```python
from build123d import *

# Parameters (mm, degrees)
SKETCH1_R           = 2.5
BOSS_EXTRUDE1_DEPTH = 6


with BuildPart() as part:
    # Sketch1 → Boss-Extrude1 (new body)
    with BuildSketch(Plane.XY):
        Polygon((140, 0), (0, 0), (0, -9), (-7, -9), (-7, -29), (0, -29), (0, -47.27), (140, -47.27), (140, -29), (147, -29), (147, -9), (140, -9), align=None)
        with Locations((120, -19)):
            Circle(SKETCH1_R, mode=Mode.SUBTRACT)
        with Locations((20, -19)):
            Circle(SKETCH1_R, mode=Mode.SUBTRACT)
        with BuildLine():
            Line((45, -34), (95, -34))
            ThreePointArc((95, -34), (110, -19), (95, -4))
            Line((95, -4), (45, -4))
            ThreePointArc((45, -4), (30, -19), (45, -34))
        make_face(mode=Mode.SUBTRACT)
    extrude(amount=BOSS_EXTRUDE1_DEPTH)


solid = part.part
```
Model file for the job. Use its own axes, mm. A direction names the side the tool comes from. Round coordinates to 2 decimals unless told otherwise and drop trailing zeros. Order: outer loops, then holes, each group sorted by start corner. A loop starts at its lowest first (then second) coordinate and runs counter-clockwise, first axis right, second up. Notation, with made-up numbers: M 73,62.5 L 132,62.5 A30 ccw 132,93.5 Z; hole C 57,48.5 d6. An arc over 180 degrees is marked long. Use CSV: the item, a comma, the result in double quotes.
Item 1: Which spindle directions (+Z, -Z, +X, -X, +Y, -Y) get a long thin tool onto all of the face, cutting with end or side? Do faces 4 (the face through (144, -9, 3)), 5 (the face through (-4, -29, 3)), 6 (the face through (140, -38, 3)), 7 (the face through (30, -19, 3)). Say none if no direction does.
Worked answers:
face 4,"+Z, -Z, +X, +Y"
face 5,"+Z, -Z, -X, -Y"
face 6,"+Z, -Z, +X, -Y"
face 7,"+Z, -Z"
Item 2: Saw through at B-B (y = -19). List the corners of the cut face in (x, z).
Worked answers:
outline,"M -7,0 L 17.5,0 L 17.5,6 L -7,6 Z; M 22.5,0 L 30,0 L 30,6 L 22.5,6 Z; M 110,0 L 117.5,0 L 117.5,6 L 110,6 Z; M 122.5,0 L 147,0 L 147,6 L 122.5,6 Z"
Item 3: Pin check, flat tips, straight feed: pin 1 (1.8 mm diameter, centred on x = -4, z = 3.5, fed in from +Y); pin 2 (1.8 mm diameter, centred on y = -41.5, z = 2, fed in from -X); pin 3 (3 mm diameter, centred on x = -3, z = 2.5, fed in from -Y). Stop position of each tip, or through.
Worked answers:
pin 1,"y = -9"
pin 2,"x = 0"
pin 3,"y = -29"
Item 4: Saw through at C-C (z = 1.5). List the corners of the cut face in (x, y).
Worked answers:
outline,"M -7,-29 L 0,-29 L 0,-47.27 L 140,-47.27 L 140,-29 L 147,-29 L 147,-9 L 140,-9 L 140,0 L 0,0 L 0,-9 L -7,-9 Z; hole C 20,-19 d5; hole M 45,-34 L 95,-34 A15 ccw 95,-4 L 45,-4 A15 ccw Z; hole C 120,-19 d5"
Item 5: Probe probe 1 along Y at (x, z) = (120, 2.15); probe 2 along X at (y, z) = (-18, 0.7); probe 3 along Y at (x, z) = (93, 1). List the from-to ranges inside material, lowest first.
Worked answers:
probe 1,"-47.27 to -21.5, -16.5 to 0"
probe 2,"-7 to 17.71, 22.29 to 30.03, 109.97 to 117.71, 122.29 to 147"
probe 3,"-47.27 to -34, -4 to 0"
Item 6: Saw through at A-A (x = 89.5). List the corners of the cut face in (y, z), plus the area to 3 significant figures.
Worked answers:
outline,"M -47.27,0 L -34,0 L -34,6 L -47.27,6 Z; M -4,0 L 0,0 L 0,6 L -4,6 Z"
area,"104 mm²"
Item 7: Saw through at D-D (y = -25.5). List the corners of the cut face in (x, z).
Worked answers:
outline,"M -7,0 L 31.48,0 L 31.48,6 L -7,6 Z; M 108.52,0 L 147,0 L 147,6 L 108.52,6 Z"
Item 8: Pull direction Y, two halves, no side cores. Call faces 1 (the face through (71, 0, 3)), 2 (the face through (70, -4, 3)), 3 (the face through (140, -5, 3)): released by +Y, released by -Y, zero draft, split by the parting line, or undercut.
Worked answers:
face 1,"released by +Y"
face 2,"undercut"
face 3,"zero draft"
